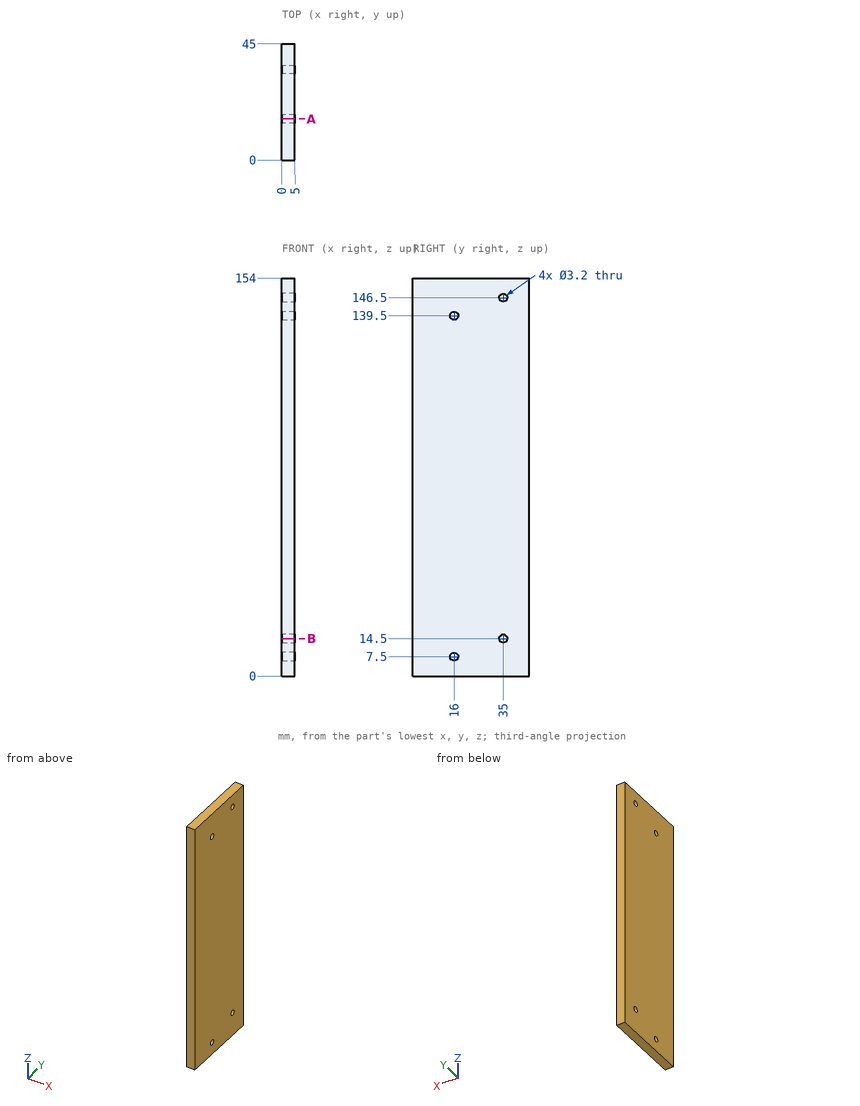
Study the drawing (mm; zero at the part's minimum x, y, z) and answer. Round coordinates to 2 decimals unless told otherwise and drop trailing zeros. Write each loop counter-clockwise with the first axis right and the second up, starting at its lowest first coordinate (ties: lowest second). Pieces come first, ordered by that corner, then holes. Notation, with made-up numbers: (-23.5, 65) -> (0.5, 65) arc R19 cw to (0.5, 91) -> close; hole circle Ø1 at (14, 17). An arc over 180 degrees is marked (long way). Write item = value, one per line.
1) Section B-B on z = 14.5 is taken. Write down the section's boundary in (x, y).
Check values:
outline = (0, 0) -> (5, 0) -> (5, 33.4) -> (0, 33.4) -> close; (0, 36.6) -> (5, 36.6) -> (5, 45) -> (0, 45) -> close
2) Section A-A on y = 16 is taken. Write down the section's boundary in (x, z), plus the area to 3 significant figures.
Check values:
outline = (0, 0) -> (5, 0) -> (5, 5.9) -> (0, 5.9) -> close; (0, 9.1) -> (5, 9.1) -> (5, 137.9) -> (0, 137.9) -> close; (0, 141.1) -> (5, 141.1) -> (5, 154) -> (0, 154) -> close
area = 738 mm²
3) Straight lines are drawn through the part: line 1 along Z through (x, y) = (1.65, 35); line 2 along Y through (x, z) = (3.8, 7.5); line 3 along Z through (x, y) = (1.25, 16). For each, find the intervals that lie inside material, in ascending order. Write a range as [from, to].
Check values:
line_1 = [0, 12.9], [16.1, 144.9], [148.1, 154]
line_2 = [0, 14.4], [17.6, 45]
line_3 = [0, 5.9], [9.1, 137.9], [141.1, 154]
4) Given pin 1 (3 mm diameter, centred on y = 35, z = 14.5, fed in from +X), flat-ended and moving along its own axis, determine where the tip first touches the part or whether it passes through.
Check values:
pin_1 = through
